Answer from the drawing. Dimensions are ordinates in mm from the lowest x, y and z of the part. A direction names the side the tool comes from. Round coordinates to 2 decimals unless told otherwise and drop trailing zeros. Loops run counter-clockwise (first coordinate to the right, second up) from the corner with the lowest first, then second, coordinate; pieces in that order, holes last.
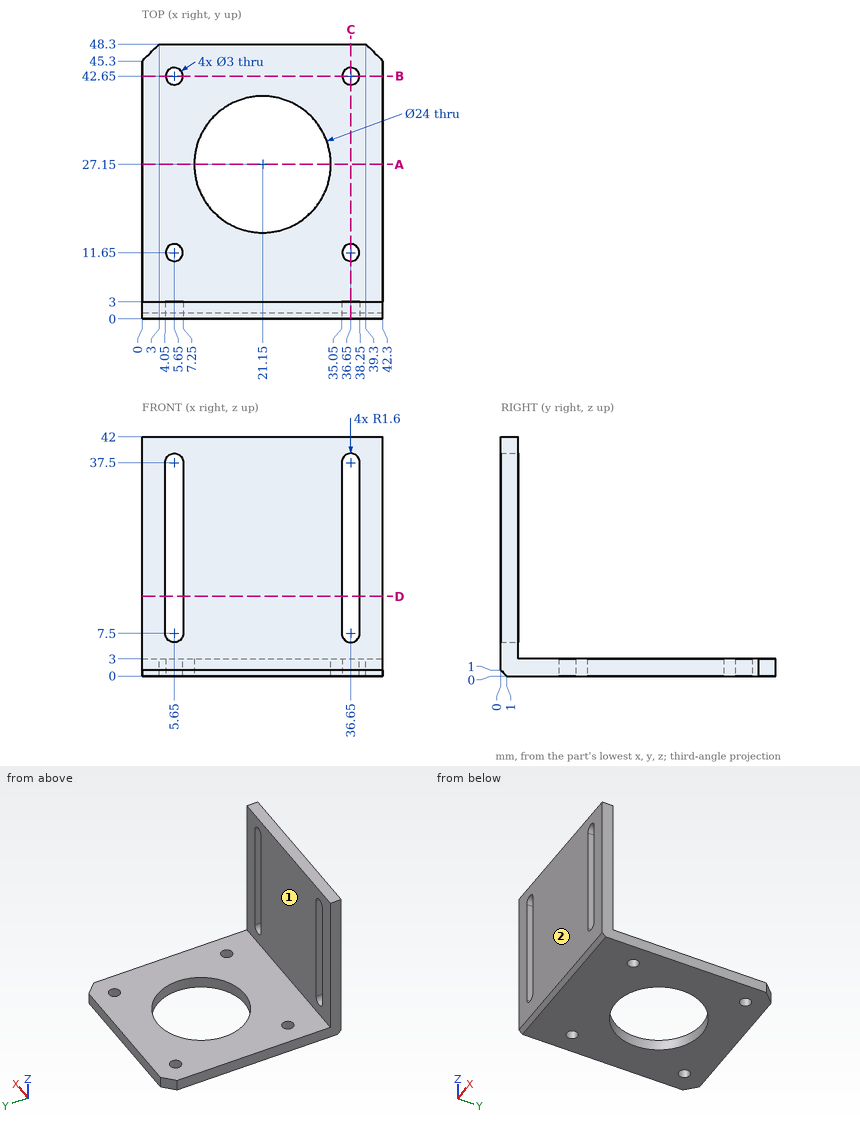
1. Find section D-D (z = 14). Write down the section's boundary in (x, y).
Answer key:
outline: (0, 0) - (4.05, 0) - (4.05, 3) - (0, 3) - close; (7.25, 0) - (35.05, 0) - (35.05, 3) - (7.25, 3) - close; (38.25, 0) - (42.3, 0) - (42.3, 3) - (38.25, 3) - close
2. Given pin 1 (1.5 mm diameter, centred on y = 1.5, z = 17.5, fed in from -X); pin 2 (5 mm diameter, centred on x = 6.5, y = 37, fed in from +Z); pin 3 (19.5 mm diameter, centred on x = 14, z = 25, fed in from +Y), each flat-ended and moving along its own axis, determine where each tip first touches the part or whether it passes through.
Answer key:
pin 1: stops at x = 0
pin 2: stops at z = 3
pin 3: stops at y = 3
3. Find section A-A (y = 27.15). Write down the section's boundary in (x, z).
Answer key:
outline: (0, 0) - (9.15, 0) - (9.15, 3) - (0, 3) - close; (33.15, 0) - (42.3, 0) - (42.3, 3) - (33.15, 3) - close
4. Consider probe 1 along Y at (x, z) = (36.65, 1.3); probe 2 along Y at (x, z) = (21, 1); probe 3 along Y at (x, z) = (36, 2). Determine where each line is inside the solid, lowest interval first.
Answer key:
probe 1: y = 0 to 10.15, 13.15 to 41.15, 44.15 to 48.3
probe 2: y = 0 to 15.15, 39.15 to 48.3
probe 3: y = 0 to 10.3, 13 to 41.3, 44 to 48.3
5. Find section C-C (x = 36.65). Write down the section's boundary in (y, z).
Answer key:
outline: (0, 1) - (1, 0) - (10.15, 0) - (10.15, 3) - (3, 3) - (3, 5.9) - (0, 5.9) - close; (0, 39.1) - (3, 39.1) - (3, 42) - (0, 42) - close; (13.15, 0) - (41.15, 0) - (41.15, 3) - (13.15, 3) - close; (44.15, 0) - (48.3, 0) - (48.3, 3) - (44.15, 3) - close
6. Find section B-B (y = 42.65). Write down the section's boundary in (x, z).
Answer key:
outline: (0, 0) - (4.15, 0) - (4.15, 3) - (0, 3) - close; (7.15, 0) - (35.15, 0) - (35.15, 3) - (7.15, 3) - close; (38.15, 0) - (42.3, 0) - (42.3, 3) - (38.15, 3) - close
7. Which of the six approach directions +Z, -Z, +X, -X, +Y, -Y give full straight-line access (tool end or side, diameter ignored) to the marked faces 1 and 2?
Answer key:
face 1: +Z, +X, -X, +Y
face 2: +Z, -Z, +X, -X, -Y
